Verification items for the finished model (mm, model axes). A direction names the side the tool comes from. Give positions to 0.01 mm unless a question says otherwise; leave off trailing zeros. Loops run counter-clockwise (first coordinate to the right, second up) from the corner with the lowest first, then second, coordinate; pieces in that order, holes last. Notation, with made-up numbers: M 68,16.5 L 95,16.5 A23 cw 95,39.5 Z; hole C 12,89.25 d10. An arc over 180 degrees is marked long. Use a Markdown table: item, result.
from build123d import *

# Parameters (mm, degrees)
SKETCH_1_R          = 2.25
SKETCH_1_R_2        = 13.5
SKETCH_1_R_3        = 1.6
SKETCH_1_R_4        = 1.55
EXTRUDE_1_DEPTH     = 6
SKETCH_2_R          = 2.25
EXTRUDE_2_DEPTH     = 6
CUT_EXTRUDE_2_DEPTH = 10


with BuildPart() as part:
    # 草图1 → 凸台-拉伸1 (new body)
    with BuildSketch(Plane.XY):
        with BuildLine():
            Line((-20.113876697, 33.24519052), (-46.760858936, 18.322520948))
            ThreePointArc((-46.760858936, 18.322520948), (-54.272689389, -11.186219731), (-24.417808219, -17.176164932))
            Line((-24.417808219, -17.176164932), (-17.260273973, -12.141356418))
            ThreePointArc((-17.260273973, -12.141356418), (0, -6.678734892), (17.260273973, -12.141356418))
            Line((17.260273973, -12.141356418), (24.417808219, -17.176164932))
            ThreePointArc((24.417808219, -17.176164932), (54.272689389, -11.186219731), (46.760858936, 18.322520948))
            Line((46.760858936, 18.322520948), (20.113876697, 33.24519052))
            ThreePointArc((20.113876697, 33.24519052), (16.372681963, 36.913582704), (15, 41.970200496))
            Line((15, 41.970200496), (15, 71.5))
            ThreePointArc((15, 71.5), (14.414213562, 72.914213562), (13, 73.5))
            Line((13, 73.5), (-13, 73.5))
            ThreePointArc((-13, 73.5), (-14.414213562, 72.914213562), (-15, 71.5))
            Line((-15, 71.5), (-15, 41.970200496))
            ThreePointArc((-15, 41.970200496), (-16.372681963, 36.913582704), (-20.113876697, 33.24519052))
        make_face()
        with Locations((-14, 27.5)):
            Circle(SKETCH_1_R, mode=Mode.SUBTRACT)
        with Locations((14, 27.5)):
            Circle(SKETCH_1_R, mode=Mode.SUBTRACT)
        with Locations((36.5, 0)):
            Circle(SKETCH_1_R_2, mode=Mode.SUBTRACT)
        with Locations((24.125631329, 12.374368671)):
            Circle(SKETCH_1_R_3, mode=Mode.SUBTRACT)
        with Locations((48.874368671, 12.374368671)):
            Circle(SKETCH_1_R_3, mode=Mode.SUBTRACT)
        with Locations((48.874368671, -12.374368671)):
            Circle(SKETCH_1_R_3, mode=Mode.SUBTRACT)
        with Locations((24.125631329, -12.374368671)):
            Circle(SKETCH_1_R_3, mode=Mode.SUBTRACT)
        Circle(SKETCH_1_R, mode=Mode.SUBTRACT)
        with Locations(Location((-24.125631329, -12.374368671, 0), (0, 0, 180))):
            Circle(SKETCH_1_R_3, mode=Mode.SUBTRACT)
        with Locations(Location((-48.874368671, -12.374368671, 0), (0, 0, 180))):
            Circle(SKETCH_1_R_3, mode=Mode.SUBTRACT)
        with Locations(Location((-48.874368671, 12.374368671, 0), (0, 0, 180))):
            Circle(SKETCH_1_R_3, mode=Mode.SUBTRACT)
        with Locations(Location((-24.125631329, 12.374368671, 0), (0, 0, 180))):
            Circle(SKETCH_1_R_3, mode=Mode.SUBTRACT)
        with Locations(Location((-36.5, 0, 0), (0, 0, 180))):
            Circle(SKETCH_1_R_2, mode=Mode.SUBTRACT)
        with Locations((-10, 37.5)):
            Circle(SKETCH_1_R_4, mode=Mode.SUBTRACT)
        with Locations((10, 37.5)):
            Circle(SKETCH_1_R_4, mode=Mode.SUBTRACT)
        with Locations((-10, 69.2)):
            Circle(SKETCH_1_R_4, mode=Mode.SUBTRACT)
        with Locations((10, 69.2)):
            Circle(SKETCH_1_R_4, mode=Mode.SUBTRACT)
        with Locations((0, 37.5)):
            Circle(SKETCH_1_R_4, mode=Mode.SUBTRACT)
    extrude(amount=EXTRUDE_1_DEPTH)

    # 草图2 → 凸台-拉伸2 (add)
    # profile 1 of 2: a face of its own
    with BuildSketch(Plane(origin=(0, 0, 0), x_dir=(-1, 0, 0), z_dir=(0, 0, -1))):
        with BuildLine():
            Line((34.034193738, -20.854730866), (72.253806486, -25.373713204))
            ThreePointArc((72.253806486, -25.373713204), (75.224328093, -24.440381608), (76.5, -21.6))
            Line((76.5, -21.6), (76.5, 3.4))
            ThreePointArc((76.5, 3.4), (75.861721596, 5.507965026), (74.16130708, 6.907788708))
            Line((74.16130708, 6.907788708), (46.760858936, 18.322520948))
            ThreePointArc((46.760858936, 18.322520948), (56.47260565, -6.488067781), (34.034193738, -20.854730866))
        make_face()
        with Locations((72.7, 3.4)):
            Circle(SKETCH_2_R, mode=Mode.SUBTRACT)
        with Locations((72.7, -21.6)):
            Circle(SKETCH_2_R, mode=Mode.SUBTRACT)
    # profile 2 of 2: a face of its own
    with BuildSketch(Plane(origin=(0, 0, 0), x_dir=(-1, 0, 0), z_dir=(0, 0, -1))):
        with BuildLine():
            Line((-74.16130708, 6.907788708), (-46.760858936, 18.322520948))
            ThreePointArc((-46.760858936, 18.322520948), (-56.47260565, -6.488067781), (-34.034193738, -20.854730866))
            Line((-34.034193738, -20.854730866), (-72.253806486, -25.373713204))
            ThreePointArc((-72.253806486, -25.373713204), (-75.224328093, -24.440381608), (-76.5, -21.6))
            Line((-76.5, -21.6), (-76.5, 3.4))
            ThreePointArc((-76.5, 3.4), (-75.861721596, 5.507965026), (-74.16130708, 6.907788708))
        make_face()
        with Locations((-72.7, 3.4)):
            Circle(SKETCH_2_R, mode=Mode.SUBTRACT)
        with Locations((-72.7, -21.6)):
            Circle(SKETCH_2_R, mode=Mode.SUBTRACT)
    extrude(amount=-EXTRUDE_2_DEPTH)

    # 草图4 → 切除-拉伸2 (cut)
    with BuildSketch(Plane(origin=(0, 0, 0), x_dir=(-1, 0, 0), z_dir=(0, 0, -1))):
        with BuildLine():
            Line((6.5, 73.5), (-6.5, 73.5))
            Line((-6.5, 73.5), (-6.5, 73))
            ThreePointArc((-6.5, 73), (-6.060660172, 71.939339828), (-5, 71.5))
            Line((-5, 71.5), (5, 71.5))
            ThreePointArc((5, 71.5), (6.060660172, 71.939339828), (6.5, 73))
            Line((6.5, 73), (6.5, 73.5))
        make_face()
    extrude(amount=-CUT_EXTRUDE_2_DEPTH, mode=Mode.SUBTRACT)


solid = part.part
(1) Cross-section at D-D on x = 30. Record the cut outline in (y, z), then the cut area to 3 significant figures.
Results below:
| item | result |
|---|---|
| outline | M -19.97,0 L -11.83,0 L -11.83,6 L -19.97,6 Z; M 11.83,0 L 27.71,0 L 27.71,6 L 11.83,6 Z |
| area | 144 mm^2 |
(2) Gauge pin test, flat ends, axial feed: P1, Ø3.5, axis at x = 14, y = 27.5, coming from the +Z side; P2, Ø4, axis at x = 10, y = 69.2, coming from the -Z side; P3, Ø3, axis at x = -36, z = 2.5, coming from the +Y side; P4, Ø2, axis at x = 11, z = 5, coming from the -Y side. Record the tip position at first contact, or that the pin passes through.
Results below:
| item | result |
|---|---|
| P1 | through |
| P2 | z = 0 |
| P3 | y = 25.19 |
| P4 | y = -9.18 |
(3) Draft check along Y on faces 3 (the cylindrical face through (75.19, -24.47, 2.96)), 4 (the cylindrical face through (9.664, 35.987, 2.958)), 5 (the flat face through (15, 57, 3)), 6 (the cylindrical face through (25.652, 12.855, 2.958)). Enter one of: +Y half, -Y half, draft (parallel to the pull), parting line (faces both ways), or undercut.
Results below:
| item | result |
|---|---|
| face 3 | -Y half |
| face 4 | undercut |
| face 5 | draft |
| face 6 | undercut |
(4) Cross-section at A-A on x = -36.5. Record the cut outline in (y, z).
Results below:
| item | result |
|---|---|
| outline | M -21.15,0 L -13.5,0 L -13.5,6 L -21.15,6 Z; M 13.5,0 L 24.07,0 L 24.07,6 L 13.5,6 Z |
(5) Material ranges on line 1 (X direction, y = 69.2, z = 2.1); line 2 (Y direction, x = 9, z = 5.1); line 3 (Y direction, x = -10, z = 4.55), recorded low to high.
Results below:
| item | result |
|---|---|
| line 1 | -15 to -11.55, -8.45 to 8.45, 11.55 to 15 |
| line 2 | -8.06 to 36.32, 38.68 to 68.02, 70.38 to 73.5 |
| line 3 | -8.39 to 35.95, 39.05 to 67.65, 70.75 to 73.5 |
(6) Cross-section at C-C on y = 61.5. Record the cut outline in (x, z), then the cut area to 3 significant figures.
Results below:
| item | result |
|---|---|
| outline | M -15,0 L 15,0 L 15,6 L -15,6 Z |
| area | 180 mm^2 |
(7) Cross-section at B-B on y = -5. Record the cut outline in (x, z).
Results below:
| item | result |
|---|---|
| outline | M -76.5,0 L -49.04,0 L -49.04,6 L -76.5,6 Z; M -23.96,0 L 23.96,0 L 23.96,6 L -23.96,6 Z; M 49.04,0 L 76.5,0 L 76.5,6 L 49.04,6 Z |
(8) Set-up check for faces 1 (the flat face through (1, 14, 0)), 2 (the cylindrical face through (-29.07, -19.64, 2.96)): record each of +Z, -Z, +X, -X, +Y, -Y from which the full face is reachable in a straight line by a thin tool's end or side.
Results below:
| item | result |
|---|---|
| face 1 | -Z, +X, -X, +Y, -Y |
| face 2 | +Z, -Z, -Y |
